Source: CAD feature listing. Evaluate the final solid. Frame: model axes, mm. A direction names the side the tool comes from. Coordinates: 2 decimals unless noted, no trailing zeros. Order: outer loops, then holes, each group sorted by start corner. A loop starts at its lowest first (then second) coordinate and runs counter-clockwise, first axis right, second up.
```python
from build123d import *

# Parameters (mm, degrees)
SKETCH1_W           = 32
SKETCH1_H           = 30.5
SKETCH1_R           = 7.5
BOSS_EXTRUDE1_DEPTH = 60
SKETCH9_R           = 7.5
BOSS_EXTRUDE3_DEPTH = 1.8
BOSS_EXTRUDE4_START = -3.6
SKETCH10_R          = 7.5
SKETCH10_R_2        = 5
BOSS_EXTRUDE4_DEPTH = 3.6
SKETCH2_R           = 3
CUT_EXTRUDE2_DEPTH  = 8
SKETCH4_R           = 4.05
BOSS_EXTRUDE2_DEPTH = 20
SKETCH6_W           = 52
SKETCH6_H           = 1
CUT_EXTRUDE4_DEPTH  = 73.249567473
SKETCH7_R           = 1.7
CUT_EXTRUDE5_DEPTH  = 71.992957397
SKETCH8_R           = 2
CUT_EXTRUDE6_DEPTH  = 71.992957397
SKETCH11_R          = 2
CUT_EXTRUDE7_DEPTH  = 71.992957397
SKETCH12_R          = 5
CUT_EXTRUDE8_DEPTH  = 72.079181268
FILLET1_R           = 1


with BuildPart() as part:
    # Sketch1 → Boss-Extrude1 (new body)
    with BuildSketch(Plane.XY):
        with Locations((0, 2.75)):
            Rectangle(SKETCH1_W, SKETCH1_H)
        Circle(SKETCH1_R, mode=Mode.SUBTRACT)
    extrude(amount=BOSS_EXTRUDE1_DEPTH)

    # Sketch9 → Boss-Extrude3 (add, symmetric)
    with BuildSketch(Plane.XY.offset(30)):
        Circle(SKETCH9_R)
    extrude(amount=BOSS_EXTRUDE3_DEPTH, both=True)

    # Sketch10 → Boss-Extrude4 (add)
    with BuildSketch(Plane.XY.offset(60).offset(BOSS_EXTRUDE4_START)):
        Circle(SKETCH10_R)
        Circle(SKETCH10_R_2, mode=Mode.SUBTRACT)
    boss_extrude4 = extrude(amount=BOSS_EXTRUDE4_DEPTH)

    # Mirror1: Boss-Extrude4 across plane
    add(boss_extrude4.mirror(Plane.XY.offset(30)))

    # Sketch2 → Cut-Extrude2 (cut)
    with BuildSketch(Plane(origin=(0, 18, 0), x_dir=(1, 0, 0), z_dir=(0, 1, 0))):
        with Locations(Location((0, -17.5, 0), (0, 0, 180))):
            Circle(SKETCH2_R)
        with Locations(Location((0, -42.5, 0), (0, 0, 180))):
            Circle(SKETCH2_R)
    extrude(amount=-CUT_EXTRUDE2_DEPTH, mode=Mode.SUBTRACT)

    # Sketch4 → Boss-Extrude2 (add)
    with BuildSketch(Plane(origin=(16, 0, 0), x_dir=(0, 0, -1), z_dir=(1, 0, 0))):
        Polygon((-60, -6), (-60, 6), (0, 6), (0, -6), (0, -12.5), (-60, -12.5), align=None)
        with Locations((-42.5, 0)):
            Circle(SKETCH4_R, mode=Mode.SUBTRACT)
        with Locations((-17.5, 0)):
            Circle(SKETCH4_R, mode=Mode.SUBTRACT)
    extrude(amount=BOSS_EXTRUDE2_DEPTH)

    # Sketch6 → Cut-Extrude4 (cut, through all)
    with BuildSketch(Plane.XY.offset(60)):
        with Locations((10, 0)):
            Rectangle(SKETCH6_W, SKETCH6_H)
    extrude(amount=-CUT_EXTRUDE4_DEPTH, mode=Mode.SUBTRACT)


with BuildPart() as cut_extrude4_kept_piece:
    # of the separate pieces the step leaves, the one the design keeps (cut_extrude4_pieces_kept)
    add(part.part.solids().sort_by_distance((-16, -12.5, 0))[0])

    # Sketch7 → Cut-Extrude5 (cut, through all)
    with BuildSketch(Plane(origin=(0, -0.5, 0), x_dir=(1, 0, 0), z_dir=(0, 1, 0))):
        with Locations(Location((-11.6, -7.5, 0), (0, 0, 270))):
            Circle(SKETCH7_R)
        with Locations(Location((-11.6, -52.5, 0), (0, 0, 270))):
            Circle(SKETCH7_R)
        with Locations(Location((12.4, -52.5, 0), (0, 0, 270))):
            Circle(SKETCH7_R)
        with Locations(Location((12.4, -7.5, 0), (0, 0, 270))):
            Circle(SKETCH7_R)
    extrude(amount=-CUT_EXTRUDE5_DEPTH, mode=Mode.SUBTRACT)

    # Sketch8 → Cut-Extrude6 (cut, through all)
    with BuildSketch(Plane(origin=(0, -0.5, 0), x_dir=(1, 0, 0), z_dir=(0, 1, 0))):
        with Locations(Location((31, -7.5, 0), (0, 0, 270))):
            Circle(SKETCH8_R)
        with Locations(Location((31, -33, 0), (0, 0, 270))):
            Circle(SKETCH8_R)
        with Locations(Location((31, -52.5, 0), (0, 0, 270))):
            Circle(SKETCH8_R)
    extrude(amount=-CUT_EXTRUDE6_DEPTH, mode=Mode.SUBTRACT)

    # Sketch11 → Cut-Extrude7 (cut, through all)
    with BuildSketch(Plane.XZ.offset(12.5)):
        with Locations(Location((26, 17.5, 0), (0, 0, 270))):
            Circle(SKETCH11_R)
        with Locations(Location((26, 42.5, 0), (0, 0, 270))):
            Circle(SKETCH11_R)
    extrude(amount=-CUT_EXTRUDE7_DEPTH, mode=Mode.SUBTRACT)

    # Sketch12 → Cut-Extrude8 (cut, through all)
    with BuildSketch(Plane.XY.offset(60)):
        Circle(SKETCH12_R)
    extrude(amount=-CUT_EXTRUDE8_DEPTH, mode=Mode.SUBTRACT)

    # Fillet1
    fillet1_edges = [cut_extrude4_kept_piece.edges().sort_by_distance(p)[0] for p in [
        (0, -5, 60),
        (-16, -6.5, 0),
        (-16, -6.5, 60),
        (20.487468593, -0.5, 60),
        (-10.487468593, -0.5, 60),
        (-4.974937186, -0.5, 58.2),
        (-10.487468593, -0.5, 0),
        (20.487468593, -0.5, 0),
        (36, -0.5, 6.740491354),
        (36, -0.5, 30),
        (36, -0.5, 53.259508646),
        (4.974937186, -0.5, 58.2),
        (-4.974937186, -0.5, 1.8),
        (4.974937186, -0.5, 1.8),
        (-16, -0.5, 30),
        (36, -6.5, 0),
        (36, -12.5, 30),
        (10, -12.5, 0),
        (36, -4.05, 17.5),
        (36, -4.05, 42.5),
        (36, -6.5, 60),
        (-16, -12.5, 30),
        (0, -5, 3.6),
        (0, -5, 0),
        (10, -12.5, 60),
        (0, -5, 56.4),
    ]]
    fillet(fillet1_edges, radius=FILLET1_R)


solid = cut_extrude4_kept_piece.part
```
1. Draft query along Z for faces 1 (the cylindrical face through (29.226, -6.416, 33.923)), 2 (the cylindrical face through (-0.16, -7.5, 15.73)), 3 (the flat face through (-16, -7, 30)), 4 (the flat face through (10, -6, 60)). Return one class per face: +Z half, -Z half, draft (parallel to the pull), parting line (faces both ways), or undercut.
2. Section query C-C, the plane x = 12.4. Output: boundary loops of the cut face in (y, z), plus the area to 3 significant figures.
3. Section query A-A, the plane z = 17.5. Output: boundary loops of the cut face in (x, y), plus the area to 3 significant figures.
4. Material intervals for line 1 along Z through (x, y) = (26, -10.5); line 2 along Z through (x, y) = (12, -5); line 3 along X through (y, z) = (-11, 7), sorted ascending.
5. Section query B-B, the plane x = 31. Output: boundary loops of the cut face in (y, z), plus the area to 3 significant figures.
6. Section query D-D, the plane y = -9. Count the separate pieces of the cut face and the enclosed holes in it, plus the area to 3 significant figures.
7. Contact query for flat-ended pins moving along their axis: P1, Ø3.5, axis at x = 26, z = 42.5, coming from the +Y side; P2, Ø1.1, axis at y = -2.5, z = 41, coming from the +X side. Output: stop coordinate, or through.
8. Access query for faces 5 (the flat face through (16, -2, 17)), 6 (the flat face through (1.1, -6.1, 56.4)), 7 (the flat face through (20, -0.5, 30)). Directions: +Z, -Z, +X, -X, +Y, -Y. A direction counts if a zero-diameter tool reaches every point of the face in a straight line with its end or side. Return the directions, or none.
Answer key:
1. face 1: undercut
1. face 2: undercut
1. face 3: draft
1. face 4: +Z half
2. outline: (-12.5, 1) arc R1 ccw to (-11.5, 0) - (-1.5, 0) arc R1 ccw to (-0.5, 1) - (-0.5, 5.8) - (-12.5, 5.8) - close; (-12.5, 9.2) - (-0.5, 9.2) - (-0.5, 50.8) - (-12.5, 50.8) - close; (-12.5, 54.2) - (-0.5, 54.2) - (-0.5, 59) arc R1 ccw to (-1.5, 60) - (-11.5, 60) arc R1 ccw to (-12.5, 59) - close
2. area: 638 mm2
3. outline: (-16, -11.5) arc R1 ccw to (-15, -12.5) - (24, -12.5) - (24, -4.05) - (16, -4.05) - (16, -0.5) - (7.48, -0.5) arc R7.5 cw to (-7.48, -0.5) - (-15, -0.5) arc R1 ccw to (-16, -1.5) - close; (28, -12.5) - (35, -12.5) arc R1 ccw to (36, -11.5) - (36, -5.05) arc R1 ccw to (35, -4.05) - (28, -4.05) - close
3. area: 437 mm2
4. line 1: z = 0 to 15.5, 19.5 to 40.5, 44.5 to 60
4. line 2: z = 0 to 5.85, 9.15 to 50.85, 54.15 to 60
4. line 3: x = -16 to -13.22, -9.98 to 10.78, 14.02 to 29.06, 32.94 to 36
5. outline: (-12.5, 1) arc R1 ccw to (-11.5, 0) - (-1.5, 0) arc R1 ccw to (-0.5, 1) - (-0.5, 5.5) - (-12.5, 5.5) - close; (-12.5, 9.5) - (-0.5, 9.5) - (-0.5, 13.48) arc R4.05 cw to (-0.5, 21.52) - (-0.5, 31) - (-12.5, 31) - close; (-12.5, 35) - (-0.5, 35) - (-0.5, 38.48) arc R4.05 cw to (-0.5, 46.52) - (-0.5, 50.5) - (-12.5, 50.5) - close; (-12.5, 54.5) - (-0.5, 54.5) - (-0.5, 59) arc R1 ccw to (-1.5, 60) - (-11.5, 60) arc R1 ccw to (-12.5, 59) - close
5. area: 532 mm2
6. separate pieces: 1
6. enclosed holes: 9
6. area: 3,020 mm2
7. P1: passes through
7. P2: stops at x = 16
8. face 5: +X, +Y
8. face 6: +Y
8. face 7: +Z, -Z, +X, -X, +Y
